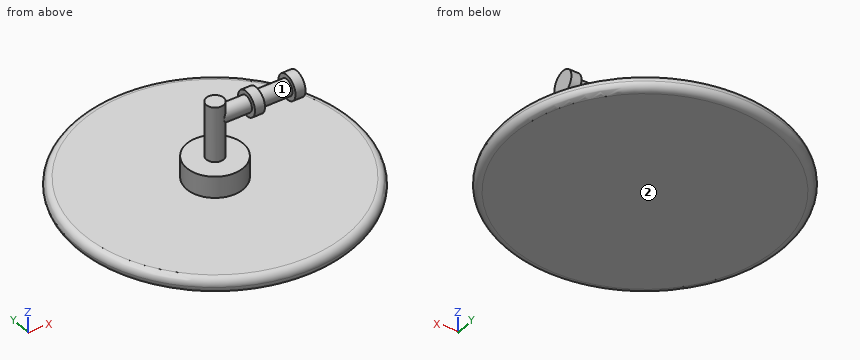
Autodesk Inventor part; units mm, degrees
ref_plane "YZ Plane" through (0, 0, 0) normal (1, 0, 0) x (0, 1, 0)
ref_plane "XZ Plane" through (0, 0, 0) normal (0, 1, 0) x (-1, 0, 0)
ref_plane "XY Plane" through (0, 0, 0) normal (0, 0, 1) x (1, 0, 0)
sketch "Sketch1" plane through (0, 0, 0) normal (0, 0, 1) x (1, 0, 0)
  circle A0 centre (0, 0) radius 203.2
  circle A1 centre (0, 0) radius 241.3
  dimension "d0" = 406.4
  dimension "d1" = 38.1
extrude "Extrusion1" add sketch "Sketch1" along normal blind 25.4 contours A0 | A1
fillet "Fillet1" radius 12.7 2 edges at (-241.3, 0, 25.4) (-241.3, 0, 0)
sketch "Sketch2" plane through (0, 0, 25.4) normal (0, 0, 1) x (1, 0, 0)
  circle A0 centre (0, 0) radius 48.9585
  dimension "d5" = 97.917
extrude "Extrusion2" add sketch "Sketch2" along normal blind 37.211
sketch "Sketch3" plane through (0, 0, 62.611) normal (0, 0, 1) x (1, 0, 0)
  circle A0 centre (0, 0) radius 14.9225
  dimension "d8" = 29.845
extrude "Extrusion3" add sketch "Sketch3" along normal blind 95.6056
sketch "Sketch5" plane through (0, 0, 0) normal (1, 0, 0) x (0, 1, 0)
  circle A0 centre (0, 131.7371) radius 13.6525
  line L0 (14.9225, 158.2166) -> (-14.9225, 158.2166)
  point P0 (0, 0)
  dimension "d11" = 27.305
  dimension "d12" = 26.4795
extrude "Extrusion4" add sketch "Sketch5" along normal blind 133.8072
sketch "Sketch6" plane through (133.8072, 0, 131.7371) normal (1, 0, 0) x (0, 0, -1)
  circle A0 centre (0, 0) radius 13.6525
  circle A1 centre (0, 0) radius 21.209
  point P0 (131.7371, 0)
  dimension "d15" = 42.418
extrude "Extrusion5" add sketch "Sketch6" against normal blind 80.4672
sketch "Sketch8" plane through (133.8072, 0, 131.7371) normal (1, 0, 0) x (0, 0, -1)
  circle A0 centre (0, 0) radius 21.209
  point P0 (131.7371, 0)
extrude "Extrusion6" cut sketch "Sketch8" against normal blind 63.5
sketch "Sketch9" plane through (70.3072, 0, 131.7371) normal (1, 0, 0) x (0, 0, -1)
  circle A0 centre (0, 0) radius 13.6525
  circle A1 centre (0, 0) radius 13.6525
  point P0 (131.7371, 0)
extrude "Extrusion7" add sketch "Sketch9" along normal blind 51.6636
sketch "Sketch10" plane through (121.9708, 0, 131.7371) normal (1, 0, 0) x (0, 0, -1)
  circle A0 centre (0, 0) radius 21.209
  point P0 (131.7371, 0)
extrude "Extrusion8" add sketch "Sketch10" along normal blind 17.018
properties part number "pizza wheel"
Work out the finished part from the listing and answer in its coordinate system (mm). Face numbers are marked on the shaded views. Round coordinates to 2 decimals unless told otherwise and drop trailing zeros. Loops run counter-clockwise (first coordinate to the right, second up) from the corner with the lowest first, then second, coordinate; pieces in that order, holes last.
(1) The part is cut by section C-C, the plane z = 38. Give the vertices of the cut face in (x, y).
Computed values:
outline: circle Ø97.92 at (0, 0)
(2) The mould has two halves that part along Z. Classify the marked faces 1 and 2: pulls with the +Z half, pulls with the -Z half, needs draft (parallel to the pull), parting line crosses it, or undercut.
Computed values:
face 1: undercut
face 2: pulls with the -Z half
(3) Find the intervals of material crossed by L1, parallel to Z at x = -140, y = 157; L2, parallel to Z at x = -38.5, y = 8; L3, parallel to Y at x = 6, z = 121, in increasing order.
Computed values:
L1: z = 0 to 25.4
L2: z = 0 to 62.61
L3: y = -13.66 to 13.66
(4) The part is cut by section D-D, the plane z = 71. Give the vertices of the cut face in (x, y) (1 decimal).
Computed values:
outline: circle Ø29.8 at (0, 0)
(5) Each of these flat-tipped pins is pushed along its axis until it touches: P1, Ø21, axis at y = 3, z = 139, coming from the +X side; P2, Ø21, axis at y = -5.5, z = 123, coming from the -X side; P3, Ø6, axis at x = -104, y = 36.5, coming from the +Z side. Where does it stop, or does it pass through?
Computed values:
P1: stops at x = 138.99
P2: stops at x = -14.92
P3: stops at z = 25.4
